```python
from build123d import *

# Parameters (mm, degrees)
ESBO_O1_W                = 150
ESBO_O1_H                = 150
RESSALTO_EXTRUS_O1_DEPTH = 50
ESBO_O2_W                = 100
ESBO_O2_H                = 30
CORTE_EXTRUS_O1_DEPTH    = 20
ESBO_O3_R                = 12.5
CORTE_EXTRUS_O2_DEPTH    = 45


with BuildPart() as part:
    # Esboço1 → Ressalto-extrusão1 (new body)
    with BuildSketch(Plane.XY):
        Rectangle(ESBO_O1_W, ESBO_O1_H)
    extrude(amount=RESSALTO_EXTRUS_O1_DEPTH)

    # Esboço2 → Corte-extrusão1 (cut)
    with BuildSketch(Plane.XY.offset(50)):
        with Locations((0, 47.564970211)):
            Rectangle(ESBO_O2_W, ESBO_O2_H)
    extrude(amount=-CORTE_EXTRUS_O1_DEPTH, mode=Mode.SUBTRACT)

    # Esboço3 → Corte-extrusão2 (cut)
    with BuildSketch(Plane.XY.offset(50)):
        with Locations((-44.493882085, -35)):
            Circle(ESBO_O3_R)
        with Locations((0, -35)):
            Circle(ESBO_O3_R)
        with Locations((45.506117915, -35)):
            Circle(ESBO_O3_R)
    extrude(amount=-CORTE_EXTRUS_O2_DEPTH, mode=Mode.SUBTRACT)


solid = part.part
```
For this review, take the finished solid that the model builds, in its own axes (mm). A direction names the side the tool comes from. Give positions to 0.01 mm unless a question says otherwise; leave off trailing zeros. Loops run counter-clockwise (first coordinate to the right, second up) from the corner with the lowest first, then second, coordinate; pieces in that order, holes last. Notation, with made-up numbers: M 9.25,52 L 43.25,52 A20 cw 43.25,64 Z; hole C 85,87 d6. An arc over 180 degrees is marked long. One line per item, written item: value. Start each with the question number.
Q1. For L1, parallel to Y at x = 0, z = 35; L2, parallel to Y at x = 0, z = 24; L3, parallel to Y at x = -34.5, z = 45.5, list the stretches that pass through material, from the lowest coordinate up.
Q2. Machinability: for faces 5 (the face through (6.72, -24.46, 27.82)), 6 (the face through (-1, 75, 25)), which of the approach directions +Z, -Z, +X, -X, +Y, -Y give a long, thin tool a straight path to every point of the face, cutting with its end or side? Answer none if there is none.
Q3. Add section C-C (x = -19.5). Give the boundary of the cut face in (y, z).
Q4. Clearance check with flat-ended pins moving along their axes: pin 1 Ø9 at (x, y) = (6.5, 49.5) entering from +Z; pin 2 Ø20 at (x, y) = (44, -36) entering from +Z. State where each tip first meets the part, or that it passes through.
Q5. Add section D-D (y = -35). Give the boundary of the cut face in (x, z).
Q6. Draft analysis for pull direction Y (two halves, no side actions). For faces 1 (the face through (-1, -75, 25)), 2 (the face through (-1, 1, 0)), 3 (the face through (52.226, -24.46, 27.815)), 4 (the face through (50, 47, 40)), state which applies: released by +Y, released by -Y, zero draft, split by the parting line, or undercut.
Q7. Add section B-B (z = 14). Give the boundary of the cut face in (x, y), and give its area (3 significant figures).
Q8. Add section A-A (z = 43.5). Give the boundary of the cut face in (x, y), and give its area (3 significant figures).
Reply:
1. L1: -75 to -47.5, -22.5 to 32.56, 62.56 to 75
1. L2: -75 to -47.5, -22.5 to 75
1. L3: -75 to -42.51, -27.49 to 32.56, 62.56 to 75
2. face 5: +Z
2. face 6: +Z, -Z, +X, -X, +Y
3. outline: M -75,0 L 75,0 L 75,50 L 62.56,50 L 62.56,30 L 32.56,30 L 32.56,50 L -75,50 Z
4. pin 1: z = 30
4. pin 2: z = 5
5. outline: M -75,0 L 75,0 L 75,50 L 58.01,50 L 58.01,5 L 33.01,5 L 33.01,50 L 12.5,50 L 12.5,5 L -12.5,5 L -12.5,50 L -31.99,50 L -31.99,5 L -56.99,5 L -56.99,50 L -75,50 Z
6. face 1: released by -Y
6. face 2: zero draft
6. face 3: undercut
6. face 4: undercut
7. outline: M -75,-75 L 75,-75 L 75,75 L -75,75 Z; hole C -44.49,-35 d25; hole C 0,-35 d25; hole C 45.51,-35 d25
7. area: 21,000 mm²
8. outline: M -75,-75 L 75,-75 L 75,75 L -75,75 Z; hole C -44.49,-35 d25; hole M -50,32.56 L 50,32.56 L 50,62.56 L -50,62.56 Z; hole C 0,-35 d25; hole C 45.51,-35 d25
8. area: 18,000 mm²
